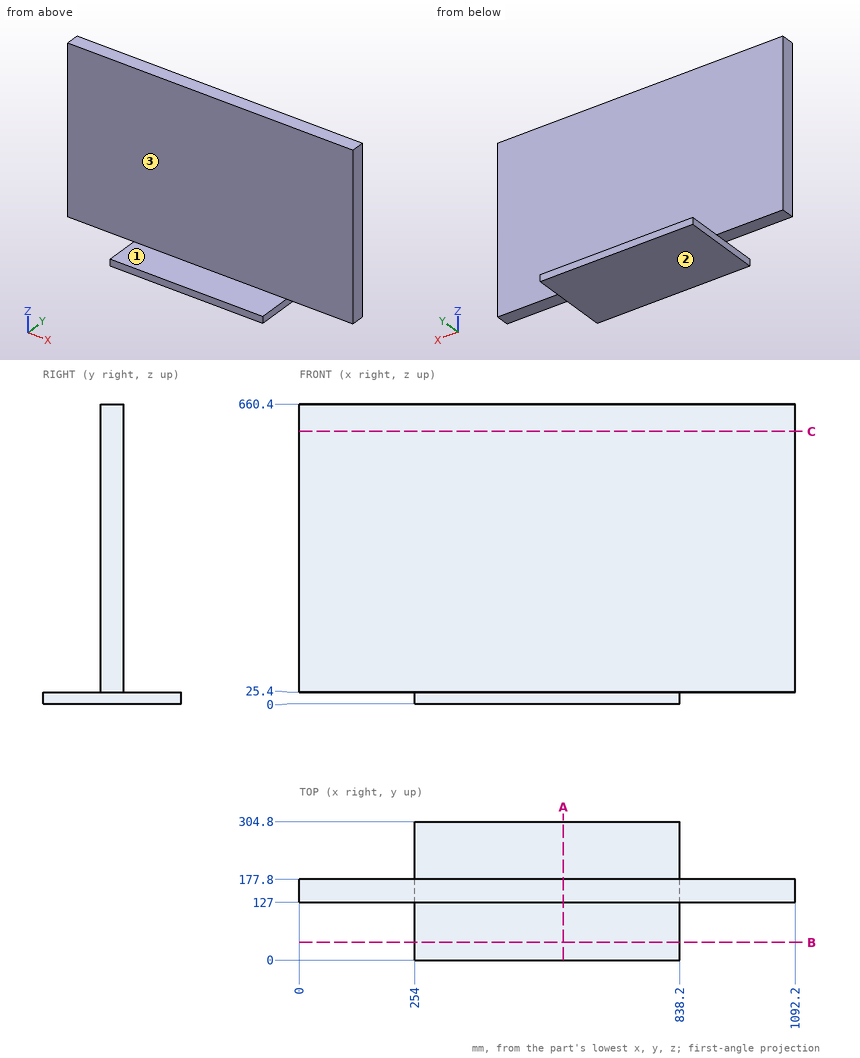
The figure shows three views and two pictorial views of one solid part (mm, origin at its lowest corner). Answer the questions. Give positions to 0.01 mm unless a question says otherwise; leave off trailing zeros. Order: outer loops, then holes, each group sorted by start corner. A loop starts at its lowest first (then second) coordinate and runs counter-clockwise, first axis right, second up. Notation, with made-up numbers: (-18, -24.5) -> (6, -24.5) arc R18 cw to (6, -13.5) -> close; hole circle Ø2 at (-18, 73). An arc over 180 degrees is marked (long way). Answer as CSV lines item,"result". Start each with the question number.
(1) Each of these flat-tipped pins is pushed along its axis until it touches: pin 1 Ø5 at (x, z) = (781.5, 200) entering from +Y; pin 2 Ø1 at (x, z) = (308.5, 99) entering from -Y; pin 3 Ø12.5 at (y, z) = (152, 12.5) entering from +X. Where does it stop, or does it pass through?
(2) Consider line 1 along Y through (x, z) = (684.5, 35); line 2 along Z through (x, y) = (751, 103); line 3 along Z through (x, y) = (1032.5, 163). Determine where each line is inside the solid, lowest interval first.
(3) Section A-A, the plane x = 582 is taken. Write down the section's boundary in (y, z).
(4) Section B-B, the plane y = 39 is taken. Write down the section's boundary in (x, z), plus the area to 3 significant figures.
(5) Section C-C, the plane z = 600 is taken. Write down the section's boundary in (x, y).
(6) For a pull along Z with two mould halves and no side action, classify the marked faces 1, 2 and 3 as released by +Z, released by -Z, zero draft, split by the parting line, or undercut.
Entries:
1,pin 1,"y = 177.8"
1,pin 2,"y = 127"
1,pin 3,"x = 838.2"
2,line 1,"127 to 177.8"
2,line 2,"0 to 25.4"
2,line 3,"25.4 to 660.4"
3,outline,"(0, 0) -> (304.8, 0) -> (304.8, 25.4) -> (177.8, 25.4) -> (177.8, 660.4) -> (127, 660.4) -> (127, 25.4) -> (0, 25.4) -> close"
4,outline,"(254, 0) -> (838.2, 0) -> (838.2, 25.4) -> (254, 25.4) -> close"
4,area,"14,800 mm²"
5,outline,"(0, 127) -> (1092.2, 127) -> (1092.2, 177.8) -> (0, 177.8) -> close"
6,face 1,"released by +Z"
6,face 2,"released by -Z"
6,face 3,"zero draft"
